Source: CAD feature listing. Evaluate the final solid. Frame: model axes, mm. A direction names the side the tool comes from. Coordinates: 2 decimals unless noted, no trailing zeros. Loops run counter-clockwise (first coordinate to the right, second up) from the corner with the lowest first, then second, coordinate; pieces in that order, holes last. Notation, with made-up numbers: M -16,51.5 L 17,51.5 A13 cw 17,59.5 Z; hole C -23,4 d5. An arc over 180 degrees is marked long. One line per question, with ' | ' between items. Start each with the question number.
1. Pin query (flat end, axial travel): P1, Ø1, axis at x = 631, y = -11.5, coming from the +Z side; P2, Ø5, axis at y = -33, z = -135.5, coming from the -X side; P3, Ø10, axis at y = -21, z = -147, coming from the +X side. Return the tip coordinate at first contact, or that it passes through.
2. Section query A-A, the plane z = -86.5. Output: boundary loops of the cut face in (x, y), and give its area (3 significant figures).
3. Section query B-B, the plane y = -21. Output: boundary loops of the cut face in (x, z).
4. Section query C-C, the plane z = -68. Output: boundary loops of the cut face in (x, y), and give its area (3 significant figures).
5. Access query for faces 5 (the flat face through (835.006, -19, -191)), 6 (the flat face through (825, -19, -177.353)). Directions: +Z, -Z, +X, -X, +Y, -Y. A direction counts if a zero-diameter tool reaches every point of the face in a straight line with its end or side. Return the directions, or none.
6. Section query D-D, the plane x = 708. Output: boundary loops of the cut face in (y, z).
7. Ray query, probe 1 along X at (y, z) = (-16, -80); probe 2 along X at (y, z) = (-22, -77); probe 3 along X at (y, z) = (-28, -177.5). Return the intervals inside material, ascending.
8. Mould query, pull axis X, two halves, no side actions, for faces 1 (the flat face through (495, -19, -177.353)), 2 (the cylindrical face through (650.081, -18.734, -117.743)), 3 (the flat face through (658, -19, -200.353)), 4 (the flat face through (787.8, -18.7, -110.5)). Classes: pulls with the +X half, pulls with the -X half, needs draft (parallel to the pull), parting line crosses it, or undercut.
```python
from build123d import *

# Parameters (mm, degrees)
F1_DEPTH = 38


# Not quite as in the source:
# - ends of sketch curves that miss each other by under 0.0002 mm in the source are joined


with BuildPart() as f1:
    # F0 (on Front) → F1 (new body)
    with BuildSketch(Plane.XZ):
        with BuildLine():
            Line((485.006122, -179.853302), (485.006122, -202.353302))
            Line((485.006122, -202.353302), (515.006122, -202.353302))
            ThreePointArc((515.006122, -202.353302), (515.5919084376, -200.9390884376), (517.006122, -200.353302))
            Line((517.006122, -200.353302), (803.006122, -200.353302))
            ThreePointArc((803.006122, -200.353302), (804.4203355624, -200.9390884376), (805.006122, -202.353302))
            Line((805.006122, -202.353302), (835.006122, -202.353302))
            Line((835.006122, -202.353302), (835.006122, -179.853302))
            Line((835.006122, -179.853302), (832.506122, -177.353302))
            Line((832.506122, -177.353302), (817.006122, -177.353302))
            ThreePointArc((817.006122, -177.353302), (815.5919084376, -176.7675155624), (815.006122, -175.353302))
            Line((815.006122, -175.353302), (815.006122, -157.353302))
            Line((815.006122, -157.353302), (759.841906, -62.353302))
            Line((759.841906, -62.353302), (737.051563, -62.353302))
            ThreePointArc((737.051563, -62.353302), (648.507993777, -117.5330565978), (579.0399418017, -39.6937430057))
            ThreePointArc((579.0399418017, -39.6937430057), (525.1590968788, -98.3321699305), (505.0179550476, -175.3772540006))
            ThreePointArc((505.0179550476, -175.3772540006), (504.4238177463, -176.7759586679), (503.018098, -177.353302))
            Line((503.018098, -177.353302), (487.506122, -177.353302))
            Line((487.506122, -177.353302), (485.006122, -179.853302))
        make_face()
    extrude(amount=F1_DEPTH)


solid = f1.part
```
Taken from the geometry:
1) P1: z = -112.79 | P2: x = 509.77 | P3: x = 811.9
2) outline: M 532.27,-38 L 595.62,-38 L 595.62,0 L 532.27,0 Z; M 724.39,-38 L 773.86,-38 L 773.86,0 L 724.39,0 Z | area: 4,290 mm^2
3) outline: M 485.01,-202.35 L 515.01,-202.35 A2 cw 517.01,-200.35 L 803.01,-200.35 A2 cw 805.01,-202.35 L 835.01,-202.35 L 835.01,-179.85 L 832.51,-177.35 L 817.01,-177.35 A2 cw 815.01,-175.35 L 815.01,-157.35 L 759.84,-62.35 L 737.05,-62.35 A81 cw 579.04,-39.69 A165 ccw 505.02,-175.38 A2 cw 503.02,-177.35 L 487.51,-177.35 L 485.01,-179.85 Z
4) outline: M 546.45,-38 L 585.03,-38 L 585.03,0 L 546.45,0 Z; M 734.98,-38 L 763.12,-38 L 763.12,0 L 734.98,0 Z | area: 2,540 mm^2
5) face 5: +Z, -Z, +X, +Y, -Y | face 6: +Z, +X, +Y, -Y
6) outline: M -38,-200.35 L 0,-200.35 L 0,-102.6 L -38,-102.6 Z
7) probe 1: 536.79 to 591.14, 728.87 to 770.09 | probe 2: 539.03 to 589.37, 730.64 to 768.35 | probe 3: 487.36 to 832.65
8) face 1: needs draft | face 2: undercut | face 3: undercut | face 4: pulls with the +X half
